Design review of the part built by this model. Coordinates are the model's own, in mm. A direction names the side the tool comes from. Give positions to 0.01 mm unless a question says otherwise; leave off trailing zeros. Loops run counter-clockwise (first coordinate to the right, second up) from the corner with the lowest first, then second, coordinate; pieces in that order, holes last. Notation, with made-up numbers: (34, -28.75) -> (81, -28.75) arc R26 cw to (81, -3.75) -> close; hole circle Ø8 at (42, 84.25). An arc over 180 degrees is marked (long way). Use a Markdown table: item, result. Add a question column.
1. Draft analysis for pull direction Z (two halves, no side actions). For faces 1 (the flat face through (-3.64, -2.61, 4.93)), 2 (the cylindrical face through (-18.523, 6.021, 8.501)), 3 (the cylindrical face through (-13.012, 5.997, 5.601)), state which applies: pulls with the +Z half, pulls with the -Z half, needs draft (parallel to the pull), parting line crosses it, or undercut.
2. To check wall thickness, follow line 1 (Z direction, x = -14.92, y = 6.05); line 2 (X direction, y = -0.75, z = 6); line 3 (X direction, y = 2, z = 6). State the ranges of each line that lie inside material, in increasing order.
3. Add section C-C (y = -1.5). State the section outline as (x, z) points.
4. Add section B-B (x = -10.25). State the section outline as (y, z) points.
5. For pin 1 Ø1.9 at (y, z) = (1.5, 4.5) entering from +X; pin 2 Ø1.3 at (y, z) = (1.5, 7) entering from -X; pin 3 Ø1.1 at (x, z) = (4, 6) entering from +Y; pin 4 Ø3.5 at (x, z) = (-14.92, 5) entering from +Y, all flat-tipped, find the tip position at first contact; note any pin that passes through.
6. Add section A-A (y = 5). State the section outline as (x, z) points.
7. For faces 4 (the flat face through (-5, -1, 5)), 5 (the flat face through (-10, 4.5, 5)), 6 (the flat face through (4, 0, 5)), 7 (the flat face through (0, -4, 5)), 8 (the flat face through (3.61, -2.64, 4.93)), list the 3-axis set-ups (+Z, -Z, +X, -X, +Y, -Y) from which the entire face can be reached by the end or side of a thin tool; tool diameter is ignored.
```python
from build123d import *

# Parameters (mm, degrees)
F1_DEPTH    = 10
F2_R        = 5.08
F3_T1_DEPTH = 28.4
F4_R        = 2
F5_DEPTH    = 25.4
F6_R        = 1.27


# Not quite as in the source:
# - a fillet or chamfer that OpenCascade refuses, or shapes differently, is made with other operations: its cross-section is extruded or revolved along the edge and cut away or added


with BuildPart() as f1:
    # F0 (on Top) → F1 (new body)
    with BuildSketch(Plane.XY):
        Polygon((-2.25, -4), (0, -4), (2.25, -4), (5, -1.25), (5, 0), (2.8, 0), (2.8, 4), (2.8, 7.5), (-20, 7.5), (-20, 4.5), (-2.8, 4.5), (-2.8, 4), (-2.8, 0), (-5, 0), (-5, -1.25), align=None)
    extrude(amount=F1_DEPTH)

    # F2
    f2_edges = [f1.edges().sort_by_distance(p)[0] for p in [
        (2.8, 7.5, 5),
    ]]
    fillet(f2_edges, radius=F2_R)

    # F3: fillet of radius 5.08 on 2 edges, made by hand

    # F3_s2 → F3_t1 (cut)
    with BuildSketch(Plane.XZ.offset(-20.2)):
        with BuildLine():
            ThreePointArc((-20, 4.92), (-18.5121024484, 8.5121024484), (-14.92, 10))
            Line((-14.92, 10), (-20, 10))
            Line((-20, 10), (-20, 4.92))
        make_face()
        with BuildLine():
            ThreePointArc((-14.92, 0), (-18.5121024484, 1.4878975516), (-20, 5.08))
            Line((-20, 5.08), (-20, 0))
            Line((-20, 0), (-14.92, 0))
        make_face()
    extrude(amount=F3_T1_DEPTH, mode=Mode.SUBTRACT)

    # F4 (on face) → F5 (cut)
    with BuildSketch(Plane.XZ.offset(-4.5)):
        with Locations((-14.92, 5)):
            Circle(F4_R)
    extrude(amount=-F5_DEPTH, mode=Mode.SUBTRACT)

    # F6
    f6_edges = [f1.edges().sort_by_distance(p)[0] for p in [
        (-16.92, 4.5, 5),
        (-16.92, 7.5, 5),
    ]]
    fillet(f6_edges, radius=F6_R)


solid = f1.part
```
Taken from the geometry:
| question | item | result |
|---|---|---|
| 1 | face 1 | needs draft |
| 1 | face 2 | pulls with the +Z half |
| 1 | face 3 | undercut |
| 2 | line 1 | z = 0 to 3, 7 to 10 |
| 2 | line 2 | x = -5 to 5 |
| 2 | line 3 | x = -2.8 to 2.8 |
| 3 | outline | (-4.75, 0) -> (4.75, 0) -> (4.75, 10) -> (-4.75, 10) -> close |
| 4 | outline | (4.5, 0) -> (7.5, 0) -> (7.5, 10) -> (4.5, 10) -> close |
| 5 | pin 1 | stops at x = 2.8 |
| 5 | pin 2 | stops at x = -2.8 |
| 5 | pin 3 | stops at y = 0 |
| 5 | pin 4 | passes through |
| 6 | outline | (-20, 5) arc R5.08 ccw to (-14.92, 0) -> (2.1, 0) -> (2.1, 10) -> (-14.92, 10) arc R5.08 ccw to start; hole circle Ø4.52 at (-14.92, 5) |
| 7 | face 4 | +Z, -Z, -X, -Y |
| 7 | face 5 | +Z, -Z, -X |
| 7 | face 6 | +Z, -Z, +X, +Y |
| 7 | face 7 | +Z, -Z, +X, -X, -Y |
| 7 | face 8 | +Z, -Z, +X, -Y |
